Geometry check sheet. Reference: drawing and pictorial views, mm from the part's lowest x, y, z. A direction names the side the tool comes from. Give positions to 0.01 mm unless a question says otherwise; leave off trailing zeros. Order: outer loops, then holes, each group sorted by start corner. A loop starts at its lowest first (then second) coordinate and runs counter-clockwise, first axis right, second up.
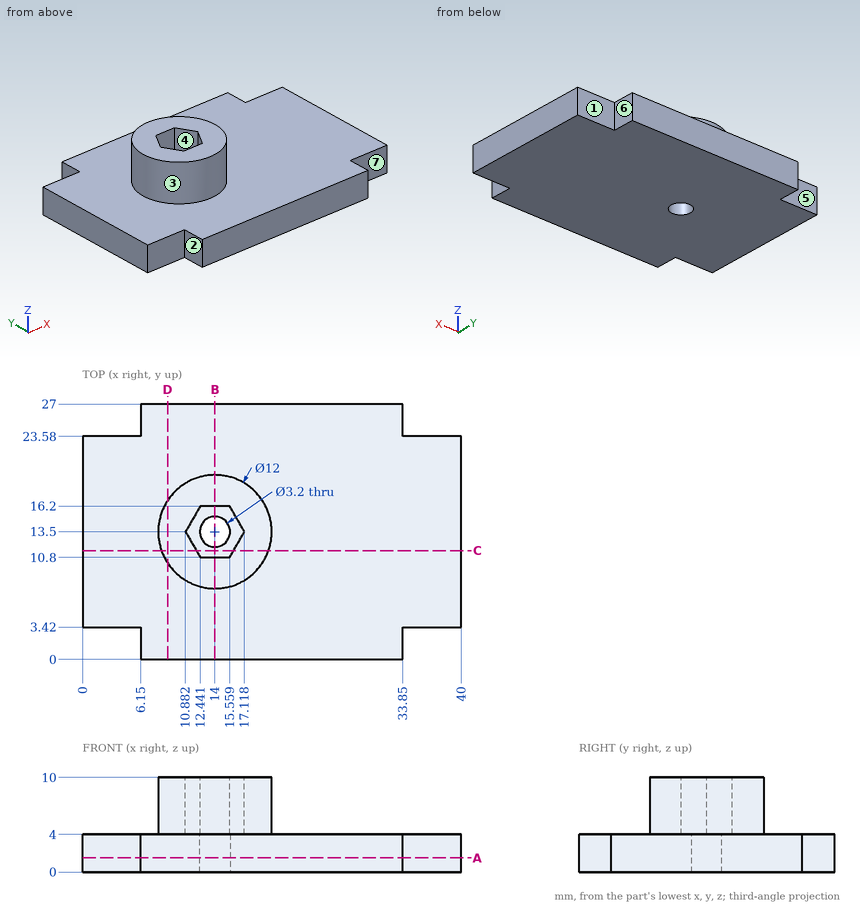
1) Section check B-B, the plane x = 14. Record the cut outline in (y, z).
Recorded:
outline: (0, 0) - (11.9, 0) - (11.9, 4) - (10.8, 4) - (10.8, 10) - (7.5, 10) - (7.5, 4) - (0, 4) - close; (15.1, 0) - (27, 0) - (27, 4) - (19.5, 4) - (19.5, 10) - (16.2, 10) - (16.2, 4) - (15.1, 4) - close
2) Material ranges on L1, parallel to Y at x = 14, z = 1.3; L2, parallel to Z at x = 13, y = 20.5; L3, parallel to X at y = 26, z = 1.25, recorded low to high.
Recorded:
L1: y = 0 to 11.9, 15.1 to 27
L2: z = 0 to 4
L3: x = 6.15 to 33.85
3) Depth check by flat-ended pin: pin 1 Ø1.7 at (y, z) = (2, 1.5) entering from +X; pin 2 Ø3 at (x, z) = (36.5, 1) entering from +Y; pin 3 Ø10 at (x, y) = (18.5, 3) entering from +Z. Enter the tip coordinate at first touch or a pass-through.
Recorded:
pin 1: stops at x = 33.85
pin 2: stops at y = 23.58
pin 3: stops at z = 4
4) Set-up check for the marked faces 1, 2 and 3: record each of +Z, -Z, +X, -X, +Y, -Y from which the full face is reachable in a straight line by a thin tool's end or side.
Recorded:
face 1: +Z, -Z, +X, +Y
face 2: +Z, -Z, -X, -Y
face 3: +Z
5) Draft check along Y on the marked faces 4, 5, 6 and 7. Enter one of: +Y half, -Y half, draft (parallel to the pull), parting line (faces both ways), or undercut.
Recorded:
face 4: undercut
face 5: +Y half
face 6: draft
face 7: -Y half
6) Section check D-D, the plane x = 9. Record the cut outline in (y, z).
Recorded:
outline: (0, 0) - (27, 0) - (27, 4) - (16.82, 4) - (16.82, 10) - (10.18, 10) - (10.18, 4) - (0, 4) - close
7) Section check A-A, the plane z = 1.5. Record the cut outline in (x, y).
Recorded:
outline: (0, 3.42) - (6.15, 3.42) - (6.15, 0) - (33.85, 0) - (33.85, 3.42) - (40, 3.42) - (40, 23.58) - (33.85, 23.58) - (33.85, 27) - (6.15, 27) - (6.15, 23.58) - (0, 23.58) - close; hole circle Ø3.2 at (14, 13.5)
8) Section check C-C, the plane y = 11.5. Record the cut outline in (x, z), then the cut area to 3 significant figures.
Recorded:
outline: (0, 0) - (40, 0) - (40, 4) - (19.66, 4) - (19.66, 10) - (15.96, 10) - (15.96, 4) - (12.04, 4) - (12.04, 10) - (8.34, 10) - (8.34, 4) - (0, 4) - close
area: 204 mm2
